Model file for the job. Use its own axes, mm. Give positions to 0.01 mm unless a question says otherwise; leave off trailing zeros. Write each loop counter-clockwise with the first axis right and the second up, starting at its lowest first coordinate (ties: lowest second). Pieces come first, ordered by that corner, then holes. Notation, with made-up numbers: (9.5, 69.25) - (46.5, 69.25) arc R24 cw to (46.5, 79.25) - close; hole circle Ø10 at (-24, 54.25). An arc over 180 degrees is marked (long way). One line per item, written item: value. Start each with the question number.
(1) Cut at B-B, the plane y = 1.9. List the corners of the cut face in (x, z), and give its area (3 significant figures).
(2) Drop flat-ended pins along their axis: P1, Ø2.5, axis at x = 9.5, y = 1.5, coming from the -Z side; P2, Ø2.5, axis at y = 1.5, z = 12.5, coming from the -X side; P3, Ø2.5, axis at x = 9, y = 1.5, coming from the -Z side. Give the stop position or say it passes through.
(3) Probe L1, parallel to Z at x = 0, y = 2.95; L2, parallel to X at y = 1.3, z = -32.5; L3, parallel to Z at x = 8, y = 0.35. List the from-to ranges inside material, lowest first.
(4) Cut at D-D, the plane z = -13. List the corners of the cut face in (x, y).
(5) Cut at C-C, the plane x = -5.25. List the corners of the cut face in (y, z), and give its area (3 significant figures).
(6) Cut at A-A, the plane x = 0. List the corners of the cut face in (y, z), and give its area (3 significant figures).
from build123d import *

# Parameters (mm, degrees)
SKETCH1_R           = 7.5
BOSS_EXTRUDE1_DEPTH = 5.08
SKETCH2_W           = 5.08
SKETCH2_H           = 15
CUT_EXTRUDE1_DEPTH  = 5.08


with BuildPart() as part:
    # Sketch1 → Boss-Extrude1 (new body)
    with BuildSketch(Plane(origin=(0, 0, 0), x_dir=(1, 0, 0), z_dir=(0, 1, 0))):
        with BuildLine():
            Line((12, -32.5), (-12, -32.5))
            Line((-12, -32.5), (-12, 32.5))
            ThreePointArc((-12, 32.5), (0, 44.5), (12, 32.5))
            Line((12, 32.5), (12, -32.5))
        make_face()
        with Locations((0, 32.5)):
            Circle(SKETCH1_R, mode=Mode.SUBTRACT)
    extrude(amount=BOSS_EXTRUDE1_DEPTH)

    # Sketch2 → Cut-Extrude1 (cut)
    with BuildSketch(Plane(origin=(0, 5.08, 0), x_dir=(1, 0, 0), z_dir=(0, 1, 0))):
        with Locations((-9.46, -15)):
            Rectangle(SKETCH2_W, SKETCH2_H)
        with Locations((-9.46, 10)):
            Rectangle(SKETCH2_W, SKETCH2_H)
    cut_extrude1 = extrude(amount=-CUT_EXTRUDE1_DEPTH, mode=Mode.SUBTRACT)

    # Mirror2: Cut-Extrude1 across plane
    add(cut_extrude1.mirror(Plane(origin=(0, 0, 0), x_dir=(0, 0, 1), z_dir=(1, 0, 0))), mode=Mode.SUBTRACT)


solid = part.part
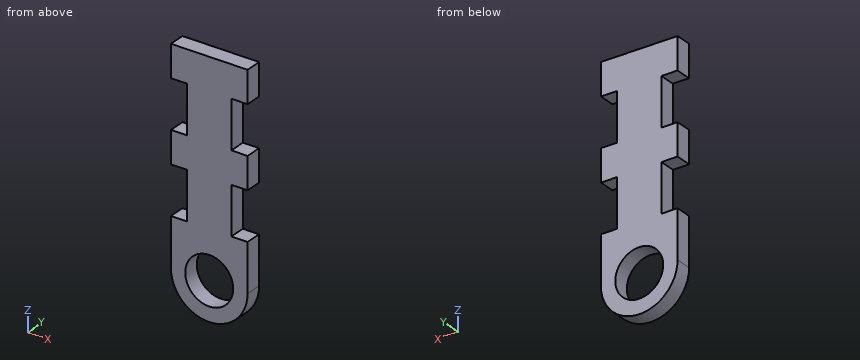
Answers follow:
1. outline: (-12, -32.5) arc R12 ccw to (12, -32.5) - (12, -17.5) - (6.92, -17.5) - (6.92, -2.5) - (12, -2.5) - (12, 7.5) - (6.92, 7.5) - (6.92, 22.5) - (12, 22.5) - (12, 32.5) - (-12, 32.5) - (-12, 22.5) - (-6.92, 22.5) - (-6.92, 7.5) - (-12, 7.5) - (-12, -2.5) - (-6.92, -2.5) - (-6.92, -17.5) - (-12, -17.5) - close; hole circle Ø15 at (0, -32.5)
1. area: 1,300 mm²
2. P1: stops at z = -41.21
2. P2: stops at x = -6.92
2. P3: stops at z = -41.66
3. L1: z = -44.5 to -40, -25 to 32.5
3. L2: x = -12 to -7.5, 7.5 to 12
3. L3: z = -41.44 to -17.5, -2.5 to 7.5, 22.5 to 32.5
4. outline: (-6.92, 0) - (6.92, 0) - (6.92, 5.08) - (-6.92, 5.08) - close
5. outline: (0, -43.29) - (5.08, -43.29) - (5.08, -37.86) - (0, -37.86) - close; (0, -27.14) - (5.08, -27.14) - (5.08, 32.5) - (0, 32.5) - close
5. area: 331 mm²
6. outline: (0, -44.5) - (5.08, -44.5) - (5.08, -40) - (0, -40) - close; (0, -25) - (5.08, -25) - (5.08, 32.5) - (0, 32.5) - close
6. area: 315 mm²
